from build123d import *

# Parameters (mm, degrees)
SKETCH1_R           = 3.5
BOSS_EXTRUDE4_DEPTH = 3


with BuildPart() as part:
    # Sketch1 → Boss-Extrude4 (new body)
    with BuildSketch(Plane.XY):
        with BuildLine():
            Line((40.907222951, 78.478335293), (40.907222951, 69.478335293))
            Line((40.907222951, 69.478335293), (36.117637198, 64.68874954))
            Line((36.117637198, 64.68874954), (-34.882362802, 64.68874954))
            Line((-34.882362802, 64.68874954), (-40.091689495, 69.898076234))
            Line((-40.091689495, 69.898076234), (-40.091689495, 78.898076234))
            ThreePointArc((-40.091689495, 78.898076234), (-49.132065099, 73.609035988), (-57.484272884, 67.288991455))
            Line((-57.484272884, 67.288991455), (-50.010639861, 61.271649914))
            Line((-50.010639861, 61.271649914), (-76.007199085, 24.540479112))
            Line((-76.007199085, 24.540479112), (-83.353433246, 29.739790957))
            ThreePointArc((-83.353433246, 29.739790957), (-88.270800728, -6.365197476), (-78.224190194, -41.391135144))
            Line((-78.224190194, -41.391135144), (-71.512419999, -35.395124733))
            Line((-71.512419999, -35.395124733), (-40.940828333, -68.415993634))
            Line((-40.940828333, -68.415993634), (-47.259115036, -74.825303514))
            ThreePointArc((-47.259115036, -74.825303514), (-0.932389989, -88.495088276), (45.672070369, -75.80443251))
            Line((45.672070369, -75.80443251), (41.027453044, -68.09550717))
            Line((41.027453044, -68.09550717), (71.689643186, -35.158748136))
            Line((71.689643186, -35.158748136), (78.276994993, -41.291186165))
            ThreePointArc((78.276994993, -41.291186165), (88.193747334, -7.356149214), (84.035885506, 27.752836742))
            Line((84.035885506, 27.752836742), (77.592312878, 23.684716135))
            Line((77.592312878, 23.684716135), (51.638414625, 60.446043171))
            Line((51.638414625, 60.446043171), (57.484272884, 67.288991455))
            ThreePointArc((57.484272884, 67.288991455), (49.512846485, 73.353445951), (40.907222951, 78.478335293))
        make_face()
        with Locations((-50.010639861, 36.027804692)):
            Circle(SKETCH1_R, mode=Mode.SUBTRACT)
        with Locations((-50.010639861, 44.965616211)):
            Circle(SKETCH1_R, mode=Mode.SUBTRACT)
        with Locations((-50.010639861, 53.137329599)):
            Circle(SKETCH1_R, mode=Mode.SUBTRACT)
        with Locations((-38.818072409, 35.897833432)):
            Circle(SKETCH1_R, mode=Mode.SUBTRACT)
        with Locations((-38.818072409, 44.835644951)):
            Circle(SKETCH1_R, mode=Mode.SUBTRACT)
        with Locations((-38.818072409, 53.007358339)):
            Circle(SKETCH1_R, mode=Mode.SUBTRACT)
        with Locations((-27.380273971, 36.073024906)):
            Circle(SKETCH1_R, mode=Mode.SUBTRACT)
        with Locations((-27.380273971, 45.010836425)):
            Circle(SKETCH1_R, mode=Mode.SUBTRACT)
        with Locations((-27.380273971, 53.182549814)):
            Circle(SKETCH1_R, mode=Mode.SUBTRACT)
        with Locations((-15.519969393, 36.039045095)):
            Circle(SKETCH1_R, mode=Mode.SUBTRACT)
        with Locations((-15.519969393, 44.976856614)):
            Circle(SKETCH1_R, mode=Mode.SUBTRACT)
        with Locations((-15.519969393, 53.148570003)):
            Circle(SKETCH1_R, mode=Mode.SUBTRACT)
        with Locations((-15.286095681, 10.286313721)):
            Circle(SKETCH1_R, mode=Mode.SUBTRACT)
        with Locations((-15.286095681, 19.22412524)):
            Circle(SKETCH1_R, mode=Mode.SUBTRACT)
        with Locations((-15.286095681, 27.395838628)):
            Circle(SKETCH1_R, mode=Mode.SUBTRACT)
        with Locations(Location((15.286095681, 27.395838628, 0), (0, 0, 180))):
            Circle(SKETCH1_R, mode=Mode.SUBTRACT)
        with Locations(Location((15.286095681, 19.22412524, 0), (0, 0, 180))):
            Circle(SKETCH1_R, mode=Mode.SUBTRACT)
        with Locations(Location((15.286095681, 10.286313721, 0), (0, 0, 180))):
            Circle(SKETCH1_R, mode=Mode.SUBTRACT)
        with Locations(Location((15.519969393, 53.148570003, 0), (0, 0, 180))):
            Circle(SKETCH1_R, mode=Mode.SUBTRACT)
        with Locations(Location((15.519969393, 44.976856614, 0), (0, 0, 180))):
            Circle(SKETCH1_R, mode=Mode.SUBTRACT)
        with Locations(Location((15.519969393, 36.039045095, 0), (0, 0, 180))):
            Circle(SKETCH1_R, mode=Mode.SUBTRACT)
        with Locations(Location((27.380273971, 53.182549814, 0), (0, 0, 180))):
            Circle(SKETCH1_R, mode=Mode.SUBTRACT)
        with Locations(Location((27.380273971, 45.010836425, 0), (0, 0, 180))):
            Circle(SKETCH1_R, mode=Mode.SUBTRACT)
        with Locations(Location((27.380273971, 36.073024906, 0), (0, 0, 180))):
            Circle(SKETCH1_R, mode=Mode.SUBTRACT)
        with Locations(Location((38.818072409, 53.007358339, 0), (0, 0, 180))):
            Circle(SKETCH1_R, mode=Mode.SUBTRACT)
        with Locations(Location((38.818072409, 44.835644951, 0), (0, 0, 180))):
            Circle(SKETCH1_R, mode=Mode.SUBTRACT)
        with Locations(Location((38.818072409, 35.897833432, 0), (0, 0, 180))):
            Circle(SKETCH1_R, mode=Mode.SUBTRACT)
        with Locations(Location((50.010639861, 53.137329599, 0), (0, 0, 180))):
            Circle(SKETCH1_R, mode=Mode.SUBTRACT)
        with Locations(Location((50.010639861, 44.965616211, 0), (0, 0, 180))):
            Circle(SKETCH1_R, mode=Mode.SUBTRACT)
        with Locations(Location((50.010639861, 36.027804692, 0), (0, 0, 180))):
            Circle(SKETCH1_R, mode=Mode.SUBTRACT)
        with Locations(Location((45.632189444, 70.091606922, 0), (0, 0, 180))):
            Circle(SKETCH1_R, mode=Mode.SUBTRACT)
        with Locations(Location((45.632189444, 61.919893534, 0), (0, 0, 180))):
            Circle(SKETCH1_R, mode=Mode.SUBTRACT)
        with Locations(Location((-44.706992882, 70.805142898, 0), (0, 0, 180))):
            Circle(SKETCH1_R, mode=Mode.SUBTRACT)
        with Locations(Location((-44.706992882, 62.633429509, 0), (0, 0, 180))):
            Circle(SKETCH1_R, mode=Mode.SUBTRACT)
        with Locations(Location((-80.683898282, 20.806109394, 0), (0, 0, 180))):
            Circle(SKETCH1_R, mode=Mode.SUBTRACT)
        with Locations(Location((-81.906376937, 11.750868753, 0), (0, 0, 180))):
            Circle(SKETCH1_R, mode=Mode.SUBTRACT)
        with Locations(Location((-82.69617398, 2.61178329, 0), (0, 0, 180))):
            Circle(SKETCH1_R, mode=Mode.SUBTRACT)
        with Locations(Location((-81.906376937, -7.043388597, 0), (0, 0, 180))):
            Circle(SKETCH1_R, mode=Mode.SUBTRACT)
        with Locations(Location((-80.683898282, -16.592800559, 0), (0, 0, 180))):
            Circle(SKETCH1_R, mode=Mode.SUBTRACT)
        with Locations(Location((-78.806996032, -24.687731454, 0), (0, 0, 180))):
            Circle(SKETCH1_R, mode=Mode.SUBTRACT)
        with Locations(Location((-76.007199085, -33.147251611, 0), (0, 0, 180))):
            Circle(SKETCH1_R, mode=Mode.SUBTRACT)
        with Locations((76.007199085, -33.147251611)):
            Circle(SKETCH1_R, mode=Mode.SUBTRACT)
        with Locations((78.806996032, -24.687731454)):
            Circle(SKETCH1_R, mode=Mode.SUBTRACT)
        with Locations((80.683898282, -16.592800559)):
            Circle(SKETCH1_R, mode=Mode.SUBTRACT)
        with Locations((81.906376937, -7.043388597)):
            Circle(SKETCH1_R, mode=Mode.SUBTRACT)
        with Locations((82.69617398, 2.61178329)):
            Circle(SKETCH1_R, mode=Mode.SUBTRACT)
        with Locations((81.906376937, 11.750868753)):
            Circle(SKETCH1_R, mode=Mode.SUBTRACT)
        with Locations((80.683898282, 20.806109394)):
            Circle(SKETCH1_R, mode=Mode.SUBTRACT)
        with Locations(Location((-34.882362802, -73.506007736, 0), (0, 0, 180))):
            Circle(SKETCH1_R, mode=Mode.SUBTRACT)
        with Locations(Location((-25.399755691, -77.973845143, 0), (0, 0, 180))):
            Circle(SKETCH1_R, mode=Mode.SUBTRACT)
        with Locations(Location((-2.136188505, -81.979492473, 0), (0, 0, 180))):
            Circle(SKETCH1_R, mode=Mode.SUBTRACT)
        with Locations(Location((0, 0, 0), (0, 0, 180))):
            Circle(SKETCH1_R, mode=Mode.SUBTRACT)
        with Locations(Location((-14.162695034, -80.592922243, 0), (0, 0, 180))):
            Circle(SKETCH1_R, mode=Mode.SUBTRACT)
        with Locations(Location((10.835227364, -80.592922243, 0), (0, 0, 180))):
            Circle(SKETCH1_R, mode=Mode.SUBTRACT)
        with Locations(Location((23.746455781, -77.973845143, 0), (0, 0, 180))):
            Circle(SKETCH1_R, mode=Mode.SUBTRACT)
        with Locations(Location((36.117637198, -73.506007736, 0), (0, 0, 180))):
            Circle(SKETCH1_R, mode=Mode.SUBTRACT)
        with BuildLine():
            Line((10.835227364, 0), (63.452114531, 39.985361841))
            ThreePointArc((63.452114531, 39.985361841), (74.999998004, -0.017304729), (63.433656153, -40.014638159))
            Line((63.433656153, -40.014638159), (10.835227364, 0))
        make_face(mode=Mode.SUBTRACT)
        with BuildLine():
            Line((0, -7.043388597), (-50.013278945, -55.889819549))
            ThreePointArc((-50.013278945, -55.889819549), (-0.017815574, -74.999997884), (49.986721055, -55.913573648))
            Line((49.986721055, -55.913573648), (0, -7.043388597))
        make_face(mode=Mode.SUBTRACT)
        with BuildLine():
            Line((-14.162695034, 0), (-63.289128306, -40.242840832))
            ThreePointArc((-63.289128306, -40.242840832), (-74.999450569, -0.287078916), (-63.59534806, 39.757159168))
            Line((-63.59534806, 39.757159168), (-14.162695034, 0))
        make_face(mode=Mode.SUBTRACT)
    extrude(amount=BOSS_EXTRUDE4_DEPTH)


solid = part.part
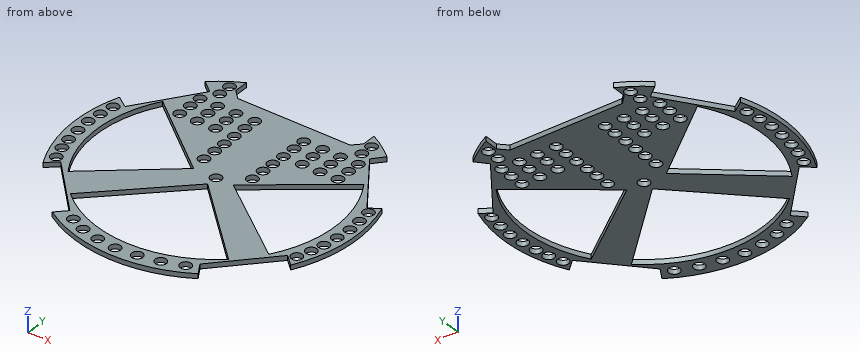
The listing builds one solid part. Answer for the finished solid, in the listing's coordinates (mm). Coordinates: 2 decimals unless noted, no trailing zeros. Order: outer loops, then holes, each group sorted by start corner. A loop starts at its lowest first (then second) coordinate and runs counter-clockwise, first axis right, second up. Notation, with made-up numbers: M 53.25,-11 L 109.25,-11 A14 ccw 109.25,-6 Z; hole C 33.5,46.25 d10. An arc over 180 degrees is marked long. Use CSV: the item, a comma, the result in double quotes.
Q1. Straight lines are drawn through the part: L1, parallel to Y at x = 29, z = 0.95; L2, parallel to Y at x = 55, z = 2.65; L3, parallel to X at y = -1, z = 1.6. For each, find the intervals that lie inside material, in ascending order.
Here are the results:
L1,"-83.61 to -69.17, -35.4 to -13.82, 13.8 to 32.97, 39.18 to 41.91, 48.11 to 50.08, 56.29 to 64.69"
L2,"-53.09 to -33.6, 33.56 to 55.68, 64.38 to 69.33"
L3,"-88.49 to -74.99, -15.38 to -3.35, 3.35 to 12.15, 74.99 to 88.49"
Q2. Section B-B (x = 67) is taken. Determine the outline of the cut face in (y, z).
Here are the results:
outline,"M -40.2,0 L -33.7,0 L -33.7,3 L -40.2,3 Z; M 33.7,0 L 38.69,0 L 38.69,3 L 33.7,3 Z"
Q3. Given pin 1 Ø1.5 at (y, z) = (-39, 2.5) entering from -X, flat-ended and moving along its own axis, determine where the tip first touches the part or whether it passes through.
Here are the results:
pin 1,"x = -79.81"
Q4. Section C-C (z = 0.7) is taken. Give the number of separate pieces and of enclosed holes in the cut face, then the cut area to 3 significant figures.
Here are the results:
separate pieces,"1"
enclosed holes,"59"
area,"9,720 mm2"
Q5. Section A-A (y = -43.5) is taken. Determine the outline of the cut face in (x, z), then the cut area to 3 significant figures.
Here are the results:
outline,"M -64.01,0 L -37.33,0 L -37.33,3 L -64.01,3 Z; M 37.29,0 L 63.92,0 L 63.92,3 L 37.29,3 Z"
area,"160 mm2"
